```python
from build123d import *

# Parameters (mm, degrees)
SKETCH_1_W          = 20
SKETCH_1_H          = 10
SKETCH_1_W_2        = 17
SKETCH_1_H_2        = 7.5
EXTRUDE_1_DEPTH     = 200
SKETCH_3_R          = 3
CUT_EXTRUDE_2_DEPTH = 10
SKETCH_5_R          = 1.5
CUT_EXTRUDE_4_DEPTH = 10
SKETCH_6_W          = 20
SKETCH_6_H          = 10
SKETCH_6_W_2        = 17
SKETCH_6_H_2        = 7.5
EXTRUDE_2_DEPTH     = 40


with BuildPart() as part:
    # 草图1 → 凸台-拉伸1 (new body)
    with BuildSketch(Plane.XY):
        Rectangle(SKETCH_1_W, SKETCH_1_H)
        Rectangle(SKETCH_1_W_2, SKETCH_1_H_2, mode=Mode.SUBTRACT)
    extrude(amount=EXTRUDE_1_DEPTH)

    # 草图3 → 切除-拉伸2 (cut)
    with BuildSketch(Plane.XZ.offset(5)):
        with Locations(Location((0, 185, 0), (0, 0, 270))):
            Circle(SKETCH_3_R)
    extrude(amount=-CUT_EXTRUDE_2_DEPTH, mode=Mode.SUBTRACT)

    # 草图5 → 切除-拉伸4 (cut)
    with BuildSketch(Plane.XZ.offset(5)):
        with Locations(Location((5.656854249, 190.656854249, 0), (0, 0, 270))):
            Circle(SKETCH_5_R)
        with Locations(Location((5.656854249, 179.343145751, 0), (0, 0, 270))):
            Circle(SKETCH_5_R)
        with Locations(Location((-5.656854249, 179.343145751, 0), (0, 0, 270))):
            Circle(SKETCH_5_R)
        with Locations(Location((-5.656854249, 190.656854249, 0), (0, 0, 270))):
            Circle(SKETCH_5_R)
    extrude(amount=-CUT_EXTRUDE_4_DEPTH, mode=Mode.SUBTRACT)

    # 草图6 → 凸台-拉伸2 (add)
    with BuildSketch(Plane(origin=(0, 0, 0), x_dir=(-1, 0, 0), z_dir=(0, 0, -1))):
        Rectangle(SKETCH_6_W, SKETCH_6_H)
        Rectangle(SKETCH_6_W_2, SKETCH_6_H_2, mode=Mode.SUBTRACT)
    extrude(amount=EXTRUDE_2_DEPTH)


solid = part.part
```
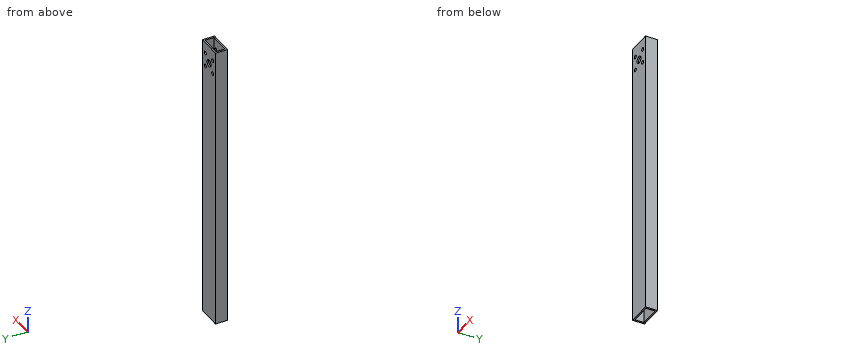
The model under review builds one solid part; all positions refer to its coordinate system, in mm. Round coordinates to 2 decimals unless told otherwise and drop trailing zeros. Loops run counter-clockwise (first coordinate to the right, second up) from the corner with the lowest first, then second, coordinate; pieces in that order, holes last. Notation, with made-up numbers: (80.25, 39.5) -> (126.25, 39.5) arc R14 ccw to (126.25, 44.5) -> close; hole circle Ø3 at (-4, 23). An arc over 180 degrees is marked (long way). Answer as a JSON object with one key per item and string values. Group by question number.
1) We need section C-C on z = 185. Write out the cut boundary in (x, y), then the cut area to 3 significant figures.
2) We need section D-D on z = 124.5. Write out the cut boundary in (x, y), then the cut area to 3 significant figures.
3) We need section A-A on y = 0.75. Write out the cut boundary in (x, z), then the cut area to 3 significant figures.
4) We need section B-B on x = 0. Write out the cut boundary in (y, z), then the cut area to 3 significant figures.
5) For line 1 (X direction, y = -2.5, z = 116.5); line 2 (Y direction, x = 0, z = 30.5); line 3 (X direction, y = -4.2, z = 185), list the stretches that pass through material, from the lowest coordinate up. Write a range as [from, to].
Result set:
{
 "1": {"outline": "(-10, -5) -> (-3, -5) -> (-3, -3.75) -> (-8.5, -3.75) -> (-8.5, 3.75) -> (-3, 3.75) -> (-3, 5) -> (-10, 5) -> close; (3, -5) -> (10, -5) -> (10, 5) -> (3, 5) -> (3, 3.75) -> (8.5, 3.75) -> (8.5, -3.75) -> (3, -3.75) -> close", "area": "57.5 mm²"},
 "2": {"outline": "(-10, -5) -> (10, -5) -> (10, 5) -> (-10, 5) -> close; hole (-8.5, -3.75) -> (8.5, -3.75) -> (8.5, 3.75) -> (-8.5, 3.75) -> close", "area": "72.5 mm²"},
 "3": {"outline": "(-10, -40) -> (-8.5, -40) -> (-8.5, 200) -> (-10, 200) -> close; (8.5, -40) -> (10, -40) -> (10, 200) -> (8.5, 200) -> close", "area": "720 mm²"},
 "4": {"outline": "(-5, -40) -> (-3.75, -40) -> (-3.75, 182) -> (-5, 182) -> close; (-5, 188) -> (-3.75, 188) -> (-3.75, 200) -> (-5, 200) -> close; (3.75, -40) -> (5, -40) -> (5, 182) -> (3.75, 182) -> close; (3.75, 188) -> (5, 188) -> (5, 200) -> (3.75, 200) -> close", "area": "585 mm²"},
 "5": {"line 1": "[-10, -8.5], [8.5, 10]", "line 2": "[-5, -3.75], [3.75, 5]", "line 3": "[-10, -3], [3, 10]"}
}
